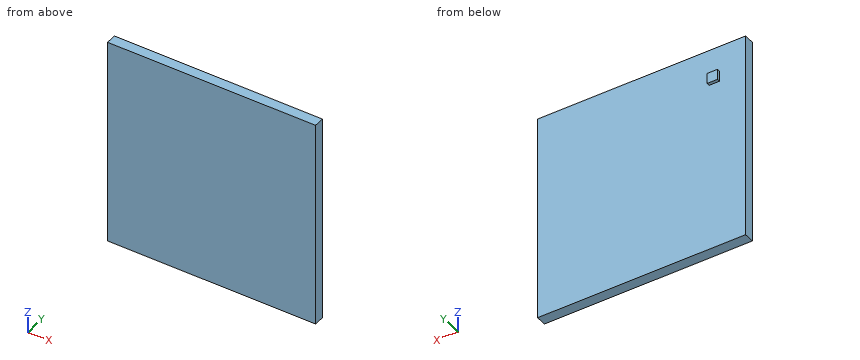
from build123d import *

# Parameters (mm, degrees)
BOSS_EXTRU_1_DEPTH = 20
ESQUISSE1_3_W      = 20
ESQUISSE1_3_H      = 20
BOSS_EXTRU_2_DEPTH = 6


with BuildPart() as part:
    # Esquisse1 → Boss.-Extru.1 (new body)
    with BuildSketch(Plane(origin=(0, 0, 0), x_dir=(1, 0, 0), z_dir=(0, 1, 0))):
        Polygon((0, 0), (200, 0), (200, 400), (-200, 400), (-200, 0), align=None)
    extrude(amount=-BOSS_EXTRU_1_DEPTH)

    # Esquisse1<3> → Boss.-Extru.2 (add)
    with BuildSketch(Plane(origin=(0, 0, 0), x_dir=(1, 0, 0), z_dir=(0, 1, 0))):
        with Locations((-140, 60)):
            Rectangle(ESQUISSE1_3_W, ESQUISSE1_3_H)
    extrude(amount=BOSS_EXTRU_2_DEPTH)


solid = part.part
Read the model definition and answer for the solid it produces. Units are mm, in the model's axes. Coordinates: 2 decimals unless noted, no trailing zeros. Order: outer loops, then holes, each group sorted by start corner. A loop starts at its lowest first (then second) coordinate and runs counter-clockwise, first axis right, second up. Notation, with made-up numbers: M 33,-3.75 L 55,-3.75 A15 cw 55,24.25 Z; hole C -27,-34.75 d7. An arc over 180 degrees is marked long. Put each result on its own line as item: value. Start each with the question number.
Item 1: Section B-B, the plane z = -111 is taken. Determine the outline of the cut face in (x, y), plus the area to 3 significant figures.
Item 2: Section A-A, the plane x = -72 is taken. Determine the outline of the cut face in (y, z), plus the area to 3 significant figures.
Item 3: Given pin 1 Ø3 at (y, z) = (2.5, -62.5) entering from -X; pin 2 Ø3 at (x, y) = (-138, 4.5) entering from +Z; pin 3 Ø3 at (y, z) = (3, -59) entering from +X, each flat-ended and moving along its own axis, determine where each tip first touches the part or whether it passes through.
Item 4: Consider probe 1 along Y at (x, z) = (-55, -118). Determine where the line is inside the solid, lowest interval first. Write a range as [from, to].
Computed:
1. outline: M -200,-20 L 200,-20 L 200,0 L -200,0 Z
1. area: 8,000 mm2
2. outline: M -20,-400 L 0,-400 L 0,0 L -20,0 Z
2. area: 8,000 mm2
3. pin 1: stops at x = -150
3. pin 2: stops at z = -50
3. pin 3: stops at x = -130
4. probe 1: y = [-20, 0]
